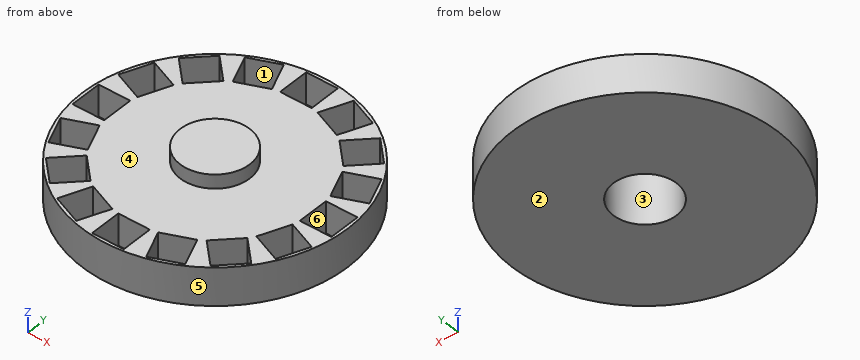
from build123d import *

# Parameters (mm, degrees)
F0_W     = 21
F0_H     = 6
F2_R     = 5
F3_DEPTH = 25
F4_W     = 5
F4_H     = 5
F5_DEPTH = 5
F2_R_2   = 5.5
F6_DEPTH = 8.2


# Not quite as in the source:
# - a feature names something its author has since deleted; it is built from what else it names


with BuildPart() as f1:
    # F0 (on Front) → F1 (revolve)
    with BuildSketch(Plane.XZ):
        with Locations((10.5, 3)):
            Rectangle(F0_W, F0_H)
    revolve(axis=Axis((0, 0, 3), (0, 0, -1)))

    # F2 (on Top) → F3 (cut)
    with BuildSketch(Plane.XY):
        Circle(F2_R)
    extrude(amount=F3_DEPTH, mode=Mode.SUBTRACT)

    # F4 (on face) → F5 (cut)
    with BuildSketch(Plane.XY.offset(6)):
        with Locations((0, 18)):
            Rectangle(F4_W, F4_H)
        Polygon((5.5353115322, 19.8962389974), (3.6218943704, 15.2768413348), (8.2412920329, 13.363424173), (10.1547091948, 17.9828218356), align=None)
        Polygon((12.7279220614, 16.2634559673), (9.1923881554, 12.7279220614), (12.7279220614, 9.1923881554), (16.2634559673, 12.7279220614), align=None)
        Polygon((17.9828218356, 10.1547091948), (13.363424173, 8.2412920329), (15.2768413348, 3.6218943704), (19.8962389974, 5.5353115322), align=None)
        with Locations((18, 0)):
            Rectangle(F4_W, F4_H)
        Polygon((19.8962389974, -5.5353115322), (15.2768413348, -3.6218943704), (13.363424173, -8.2412920329), (17.9828218356, -10.1547091948), align=None)
        Polygon((16.2634559673, -12.7279220614), (12.7279220614, -9.1923881554), (9.1923881554, -12.7279220614), (12.7279220614, -16.2634559673), align=None)
        Polygon((10.1547091948, -17.9828218356), (8.2412920329, -13.363424173), (3.6218943704, -15.2768413348), (5.5353115322, -19.8962389974), align=None)
        with Locations((0, -18)):
            Rectangle(F4_W, F4_H)
        Polygon((-5.5353115322, -19.8962389974), (-3.6218943704, -15.2768413348), (-8.2412920329, -13.363424173), (-10.1547091948, -17.9828218356), align=None)
        Polygon((-12.7279220614, -16.2634559673), (-9.1923881554, -12.7279220614), (-12.7279220614, -9.1923881554), (-16.2634559673, -12.7279220614), align=None)
        Polygon((-17.9828218356, -10.1547091948), (-13.363424173, -8.2412920329), (-15.2768413348, -3.6218943704), (-19.8962389974, -5.5353115322), align=None)
        with Locations((-18, 0)):
            Rectangle(F4_W, F4_H)
        Polygon((-19.8962389974, 5.5353115322), (-15.2768413348, 3.6218943704), (-13.363424173, 8.2412920329), (-17.9828218356, 10.1547091948), align=None)
        Polygon((-16.2634559673, 12.7279220614), (-12.7279220614, 9.1923881554), (-9.1923881554, 12.7279220614), (-12.7279220614, 16.2634559673), align=None)
        Polygon((-10.1547091948, 17.9828218356), (-8.2412920329, 13.363424173), (-3.6218943704, 15.2768413348), (-5.5353115322, 19.8962389974), align=None)
    extrude(amount=-F5_DEPTH, mode=Mode.SUBTRACT)

    # F2 (on Top) → F6 (join)
    with BuildSketch(Plane.XY):
        Circle(F2_R_2)
        Circle(F2_R, mode=Mode.SUBTRACT)
    extrude(amount=F6_DEPTH)

    # F7 (on Right) → F8 (revolve)
    with BuildSketch(Plane.YZ):
        Polygon((0, 8.2), (0, 8), (5.5, 8), (5.5, 8.2), (5.4786731489, 8.2), align=None)
    revolve(axis=Axis((0, 0, 8.1), (0, 0, -1)))


solid = f1.part
Verification items for the finished model (mm, model axes). Face numbers are marked on the shaded views. A direction names the side the tool comes from. Coordinates: 2 decimals unless noted, no trailing zeros. Loops run counter-clockwise (first coordinate to the right, second up) from the corner with the lowest first, then second, coordinate; pieces in that order, holes last. Notation, with made-up numbers: (64.25, 2.25) -> (122.25, 2.25) arc R26 cw to (122.25, 37.25) -> close; hole circle Ø10 at (29, 48.5). An arc over 180 degrees is marked (long way). Answer as a JSON object with one key per item and string values. Group by question number.
Item 1: Depth check by flat-ended pin: pin 1 (1.5 mm diameter, centred on x = -17.5, z = 4.5, fed in from +Y); pin 2 (8 mm diameter, centred on x = -14, y = 16.5, fed in from +Z); pin 3 (2 mm diameter, centred on x = 12.5, y = -13, fed in from +Z). Enter the tip coordinate at first touch or a pass-through.
Item 2: Tool access check on the marked faces 1, 2 and 3. Record the directions out of +Z, -Z, +X, -X, +Y, -Y that give a thin tool (end or side, any length) a straight path to the whole face; none if there is none.
Item 3: Sectioned sample at A-A on y = 0. Record the boundary of the cut face in (x, z), plus the area to 3 significant figures.
Item 4: Sectioned sample at C-C on z = 1.5. State how many separate pieces and enclosed holes the cut face has, plus the area to 3 significant figures.
Item 5: Mould release check, pull along Y, two halves, no side actions. Record for the marked faces 4, 5 and 6: +Y half, -Y half, draft (parallel to the pull), parting line (faces both ways), or undercut.
Item 6: Sectioned sample at D-D on z = 7. Record the boundary of the cut face in (x, y).
Item 7: Scan lines: probe 1 along X at (y, z) = (0, 3); probe 2 along X at (y, z) = (19, 5.5). Record each from-to range of solid material in increasing order.
Evaluation:
{
 "1": {"pin 1": "stops at y = 12.67", "pin 2": "stops at z = 6", "pin 3": "stops at z = 1"},
 "2": {"face 1": "+Z", "face 2": "-Z, +X, -X, +Y, -Y", "face 3": "-Z"},
 "3": {"outline": "(-21, 0) -> (-5, 0) -> (-5, 8) -> (5, 8) -> (5, 0) -> (21, 0) -> (21, 6) -> (20.5, 6) -> (20.5, 1) -> (15.5, 1) -> (15.5, 6) -> (5.5, 6) -> (5.5, 8.2) -> (-5.5, 8.2) -> (-5.5, 6) -> (-15.5, 6) -> (-15.5, 1) -> (-20.5, 1) -> (-20.5, 6) -> (-21, 6) -> close", "area": "146 mm²"},
 "4": {"separate pieces": "1", "enclosed holes": "17", "area": "907 mm²"},
 "5": {"face 4": "draft", "face 5": "parting line", "face 6": "undercut"},
 "6": {"outline": "circle Ø11 at (0, 0); hole circle Ø10 at (0, 0)"},
 "7": {"probe 1": "x = -21 to -20.5, -15.5 to -5, 5 to 15.5, 20.5 to 21", "probe 2": "x = -8.94 to -7.7, -5.16 to -2.5, 2.5 to 5.16, 7.7 to 8.94"}
}
